```python
from build123d import *

# Parameters (mm, degrees)
SKICA1_W                 = 150
SKICA1_H                 = 20
P_IDAT_VYSUNUT_M1_DEPTH  = 60
SKICA2_W                 = 110
SKICA2_H                 = 40
ODEBRAT_VYSUNUT_M1_DEPTH = 60
ZAOBLIT1_R               = 10
ZAOBLIT2_R               = 30
ZAOBLIT3_R               = 5


with BuildPart() as part:
    # Skica1 → Přidat vysunutím1 (new body)
    with BuildSketch(Plane(origin=(0, 0, 0), x_dir=(1, 0, 0), z_dir=(0, 1, 0))):
        Rectangle(SKICA1_W, SKICA1_H)
    extrude(amount=P_IDAT_VYSUNUT_M1_DEPTH)

    # Skica2 → Odebrat vysunutím1 (cut)
    with BuildSketch(Plane.XY.offset(10)):
        with Locations((0, 20)):
            Rectangle(SKICA2_W, SKICA2_H)
    extrude(amount=-ODEBRAT_VYSUNUT_M1_DEPTH, mode=Mode.SUBTRACT)

    # Zaoblit1
    zaoblit1_edges = [part.edges().sort_by_distance(p)[0] for p in [
        (-55, 40, 0),
        (55, 40, 0),
    ]]
    fillet(zaoblit1_edges, radius=ZAOBLIT1_R)

    # Zaoblit2
    zaoblit2_edges = [part.edges().sort_by_distance(p)[0] for p in [
        (75, 60, 0),
        (-75, 60, 0),
    ]]
    fillet(zaoblit2_edges, radius=ZAOBLIT2_R)

    # Zaoblit3
    zaoblit3_edges = [part.edges().sort_by_distance(p)[0] for p in [
        (55, 15, -10),
        (55, 15, 10),
        (0, 40, 10),
        (0, 40, -10),
        (-55, 15, 10),
        (-55, 15, -10),
        (52.071067812, 37.071067812, 10),
        (52.071067812, 37.071067812, -10),
        (-52.071067812, 37.071067812, 10),
        (-52.071067812, 37.071067812, -10),
        (0, 60, 10),
        (0, 60, -10),
        (-75, 15, -10),
        (75, 15, -10),
        (-66.213203436, 51.213203436, -10),
        (66.213203436, 51.213203436, -10),
        (75, 15, 10),
        (-75, 15, 10),
        (-66.213203436, 51.213203436, 10),
        (66.213203436, 51.213203436, 10),
    ]]
    fillet(zaoblit3_edges, radius=ZAOBLIT3_R)


solid = part.part
```
Design review of the part built by this model. Coordinates are the model's own, in mm. A direction names the side the tool comes from. Round coordinates to 2 decimals unless told otherwise and drop trailing zeros. Order: outer loops, then holes, each group sorted by start corner. A loop starts at its lowest first (then second) coordinate and runs counter-clockwise, first axis right, second up. Notation, with made-up numbers: M 82.25,83.25 L 91.25,83.25 A7 cw 91.25,94.25 Z; hole C -5,86 d10. An arc over 180 degrees is marked long. Put each result on its own line as item: value.
Q1. Consider section C-C (x = 32.5). State the section outline as (y, z) points, and give its area (3 significant figures).
Reported:
outline: M 40,-5 A5 ccw 45,-10 L 55,-10 A5 ccw 60,-5 L 60,5 A5 ccw 55,10 L 45,10 A5 ccw 40,5 Z
area: 379 mm²
Q2. Consider section B-B (z = 2.75). State the section outline as (x, y) points, and give its area (3 significant figures).
Reported:
outline: M -75,0 L -55,0 L -55,30 A10 cw -45,40 L 45,40 A10 cw 55,30 L 55,0 L 75,0 L 75,30 A30 ccw 45,60 L -45,60 A30 ccw -75,30 Z
area: 4,260 mm²
Q3. Machinability: for faces 4 (the face through (-56, 15, -8)), 5 (the face through (-65, 0, 0)), 6 (the face through (-57, 15, 9)), 7 (the face through (-73, 15, 9)), 8 (the face through (51.99, 37.15, -0.07)), which of the approach directions +Z, -Z, +X, -X, +Y, -Y give a long, thin tool a straight path to every point of the face, cutting with its end or side? Answer none if there is none.
Reported:
face 4: -Z, -Y
face 5: +Z, -Z, +X, -X, -Y
face 6: +Z, -Y
face 7: +Z, -X, +Y, -Y
face 8: +Z, -Z, -Y
Q4. Draft analysis for pull direction X (two halves, no side actions). For faces 1 (the face through (65.979, 51.445, -0.07)), 2 (the face through (-1, 45.4, -10)), 3 (the face through (-1, 40, 0)), state which applies: released by +X, released by -X, zero draft, split by the parting line, or undercut.
Reported:
face 1: released by +X
face 2: zero draft
face 3: undercut
Q5. To check wall thickness, follow line 1 (X direction, y = 4.5, z = 1); line 2 (Y direction, x = 22, z = -3); line 3 (Z direction, x = 19.5, y = 44.5). State the ranges of each line that lie inside material, in increasing order.
Reported:
line 1: -75 to -55, 55 to 75
line 2: 40 to 60
line 3: -9.97 to 9.97
Q6. Consider section D-D (z = -8.5). State the section outline as (x, y) points, and give its area (3 significant figures).
Reported:
outline: M -73.57,0 L -56.43,0 L -56.43,30 A11.43 cw -45,41.43 L 45,41.43 A11.43 cw 56.43,30 L 56.43,0 L 73.57,0 L 73.57,30 A28.57 ccw 45,58.57 L -45,58.57 A28.57 ccw -73.57,30 Z
area: 3,650 mm²
Q7. Consider section A-A (y = 28.5). State the section outline as (x, z) points.
Reported:
outline: M -75,-5 A5 ccw -70,-10 L -60,-10 A5 ccw -55,-5 L -55,5 A5 ccw -60,10 L -70,10 A5 ccw -75,5 Z; M 55,-5 A5 ccw 60,-10 L 70,-10 A5 ccw 75,-5 L 75,5 A5 ccw 70,10 L 60,10 A5 ccw 55,5 Z
Q8. Insertion check: pin 1 Ø10 at (x, z) = (-12, 2) entering from -Y. The pin has a flat end and moves straight along its axis. Give the tip position at first contact, or say it passes through.
Reported:
pin 1: y = 40
